Check sheet for the modelled part. Datum: model origin and axes. Units: mm. A direction names the side the tool comes from. Round coordinates to 2 decimals unless told otherwise and drop trailing zeros. Loops run counter-clockwise (first coordinate to the right, second up) from the corner with the lowest first, then second, coordinate; pieces in that order, holes last. Notation, with made-up numbers: (18, 0.5) -> (67, 0.5) arc R24 cw to (67, 13.5) -> close; hole circle Ø3 at (19, 10). An arc over 180 degrees is marked (long way). Return JSON: item names as keys, results as strings.
from build123d import *

# Parameters (mm, degrees)
F0_R     = 11
F1_DEPTH = 6


with BuildPart() as f1:
    # F0 (on Top) → F1 (new body)
    with BuildSketch(Plane.XY):
        with BuildLine():
            Line((11.2187429189, 11.8292181419), (3.5389187623, 33.7403846154))
            ThreePointArc((3.5389187623, 33.7403846154), (0, 36.25), (-3.5389187623, 33.7403846154))
            Line((-3.5389187623, 33.7403846154), (-11.2187429189, 11.8292181419))
            ThreePointArc((-11.2187429189, 11.8292181419), (-13.1608995727, 7.5984489111), (-15.8537748772, 3.8011072954))
            Line((-15.8537748772, 3.8011072954), (-30.9894895915, -13.8053987576))
            ThreePointArc((-30.9894895915, -13.8053987576), (-28.3703151015, -12.5067254343), (-25.6147048476, -13.4830653025))
            ThreePointArc((-25.6147048476, -13.4830653025), (-24.8982303588, -14.375), (-24.4840294966, -15.4414524572))
            ThreePointArc((-24.4840294966, -15.4414524572), (-24.4179418082, -15.8433278187), (-24.395825623, -16.25))
            ThreePointArc((-24.395825623, -16.25), (-25.2588111204, -18.643250355), (-27.4505708292, -19.9349858577))
            Line((-27.4505708292, -19.9349858577), (-4.6350319583, -15.6303254372))
            ThreePointArc((-4.6350319583, -15.6303254372), (0, -15.1968978222), (4.6350319583, -15.6303254372))
            Line((4.6350319583, -15.6303254372), (27.4505708292, -19.9349858577))
            ThreePointArc((27.4505708292, -19.9349858577), (25.016299495, -18.3160508741), (24.4840294966, -15.4414524572))
            ThreePointArc((24.4840294966, -15.4414524572), (24.8982303588, -14.375), (25.6147048476, -13.4830653025))
            ThreePointArc((25.6147048476, -13.4830653025), (28.3703151015, -12.5067254343), (30.9894895915, -13.8053987576))
            Line((30.9894895915, -13.8053987576), (15.8537748772, 3.8011072954))
            ThreePointArc((15.8537748772, 3.8011072954), (13.1608995727, 7.5984489111), (11.2187429189, 11.8292181419))
        make_face()
        with BuildLine():
            Line((-19.4313725784, -12.3734087272), (-12.0274698164, -8.0987634745))
            ThreePointArc((-12.0274698164, -8.0987634745), (-10.1599093098, -10.3453488494), (-7.8799155315, -12.171973185))
            Line((-7.8799155315, -12.171973185), (-18.7459713, -14.2220970264))
            ThreePointArc((-18.7459713, -14.2220970264), (-19.8690053401, -13.5870615238), (-19.4313725784, -12.3734087272))
        make_face(mode=Mode.SUBTRACT)
        with BuildLine():
            ThreePointArc((-20.4313725784, -10.6413579197), (-21.7012431124, -10.4135326105), (-21.68968297, -9.1234388512))
            Line((-21.68968297, -9.1234388512), (-14.4811957581, -0.7382204374))
            ThreePointArc((-14.4811957581, -0.7382204374), (-14.0392895695, -3.6260651377), (-13.0274698164, -6.366712667))
            Line((-13.0274698164, -6.366712667), (-20.4313725784, -10.6413579197))
        make_face(mode=Mode.SUBTRACT)
        with BuildLine():
            ThreePointArc((19.4313725784, -12.3734087272), (19.8690053401, -13.5870615238), (18.7459713, -14.2220970264))
            Line((18.7459713, -14.2220970264), (7.8799155315, -12.171973185))
            ThreePointArc((7.8799155315, -12.171973185), (10.1599093098, -10.3453488494), (12.0274698164, -8.0987634745))
            Line((12.0274698164, -8.0987634745), (19.4313725784, -12.3734087272))
        make_face(mode=Mode.SUBTRACT)
        Circle(F0_R, mode=Mode.SUBTRACT)
        with BuildLine():
            Line((14.4811957581, -0.7382204374), (21.68968297, -9.1234388512))
            ThreePointArc((21.68968297, -9.1234388512), (21.7012431124, -10.4135326105), (20.4313725784, -10.6413579197))
            Line((20.4313725784, -10.6413579197), (13.0274698164, -6.366712667))
            ThreePointArc((13.0274698164, -6.366712667), (14.0392895695, -3.6260651377), (14.4811957581, -0.7382204374))
        make_face(mode=Mode.SUBTRACT)
        with BuildLine():
            Line((-6.6012802267, 12.9101936225), (-2.9437116699, 23.3455358777))
            ThreePointArc((-2.9437116699, 23.3455358777), (-1.8322377723, 24.0005941343), (-1, 23.0147666469))
            Line((-1, 23.0147666469), (-1, 14.4654761415))
            ThreePointArc((-1, 14.4654761415), (-3.8793802597, 13.9714139872), (-6.6012802267, 12.9101936225))
        make_face(mode=Mode.SUBTRACT)
        with BuildLine():
            ThreePointArc((1, 23.0147666469), (1.8322377723, 24.0005941343), (2.9437116699, 23.3455358777))
            Line((2.9437116699, 23.3455358777), (6.6012802267, 12.9101936225))
            ThreePointArc((6.6012802267, 12.9101936225), (3.8793802597, 13.9714139872), (1, 14.4654761415))
            Line((1, 14.4654761415), (1, 23.0147666469))
        make_face(mode=Mode.SUBTRACT)
        with BuildLine():
            ThreePointArc((-25.6147048476, -13.4830653025), (-28.3703151015, -12.5067254343), (-30.9894895915, -13.8053987576))
            ThreePointArc((-30.9894895915, -13.8053987576), (-31.3934208872, -18.125), (-27.4505708292, -19.9349858577))
            ThreePointArc((-27.4505708292, -19.9349858577), (-25.2588111204, -18.643250355), (-24.395825623, -16.25))
            ThreePointArc((-24.395825623, -16.25), (-24.4179418082, -15.8433278187), (-24.4840294966, -15.4414524572))
            ThreePointArc((-24.4840294966, -15.4414524572), (-24.8982303588, -14.375), (-25.6147048476, -13.4830653025))
        make_face()
        with BuildLine():
            ThreePointArc((31.895825623, -16.25), (31.6619484793, -14.9463972771), (30.9894895915, -13.8053987576))
            ThreePointArc((30.9894895915, -13.8053987576), (28.3703151015, -12.5067254343), (25.6147048476, -13.4830653025))
            ThreePointArc((25.6147048476, -13.4830653025), (24.8982303588, -14.375), (24.4840294966, -15.4414524572))
            ThreePointArc((24.4840294966, -15.4414524572), (25.016299495, -18.3160508741), (27.4505708292, -19.9349858577))
            ThreePointArc((27.4505708292, -19.9349858577), (30.539075978, -19.1370145026), (31.895825623, -16.25))
        make_face()
    extrude(amount=F1_DEPTH)


solid = f1.part
Q1. Section check A-A (x = 0). Record the boundary of the cut face in (y, z).
Results list:
{"outline": "(-15.2, 0) -> (-11, 0) -> (-11, 6) -> (-15.2, 6) -> close; (11, 0) -> (36.25, 0) -> (36.25, 6) -> (11, 6) -> close"}
Q2. Draft check along X on faces 1 (the cylindrical face through (13.194, 7.542, 2.958)), 2 (the cylindrical face through (-1.852, 24.004, 2.958)), 3 (the flat face through (-7.325, 22.938, 2.958)). Enter one of: released by +X, released by -X, zero draft, split by the parting line, or undercut.
Results list:
{"face 1": "released by +X", "face 2": "undercut", "face 3": "released by -X"}
Q3. Tool access check on faces 4 (the flat face through (15.88, -17.75, 2.96)), 5 (the cylindrical face through (-19.86, -13.61, 2.96)), 6 (the flat face through (23.53, -5.13, 2.96)). Record the directions out of +Z, -Z, +X, -X, +Y, -Y that give a thin tool (end or side, any length) a straight path to the whole face; none if there is none.
Results list:
{"face 4": "+Z, -Z, -Y", "face 5": "+Z, -Z", "face 6": "+Z, -Z, +X, +Y"}
Q4. Go/stop test with flat-tipped pins: pin 1 (1.5 mm diameter, centred on y = 29.5, z = 5.5, fed in from -X); pin 2 (1 mm diameter, centred on x = 13, z = 4.5, fed in from -Y); pin 3 (17.5 mm diameter, centred on x = 0, y = 0, fed in from -Z). Record where each tip stops, or that it passes through.
Results list:
{"pin 1": "x = -5.29", "pin 2": "y = -17.3", "pin 3": "through"}
Q5. Section check D-D (y = 25). Record the boundary of the cut face in (x, z).
Results list:
{"outline": "(-6.6, 0) -> (6.6, 0) -> (6.6, 6) -> (-6.6, 6) -> close"}
Q6. Section check C-C (z = 5.1). Count the separate pieces of the cut face and the enclosed holes in it, then the cut area to 3 significant figures.
Results list:
{"separate pieces": "1", "enclosed holes": "7", "area": "1,030 mm^2"}
Q7. Material ranges on line 1 (Y direction, x = 0, z = 1.7); line 2 (X direction, y = 18, z = 3.5); line 3 (X direction, y = -4.5, z = 2.15), recorded low to high.
Results list:
{"line 1": "-15.2 to -11, 11 to 36.25", "line 2": "-9.06 to -4.82, -1 to 1, 4.82 to 9.06", "line 3": "-22.99 to -17.72, -13.78 to -10.04, 10.04 to 13.78, 17.72 to 22.99"}
Q8. Section check B-B (y = 0). Record the boundary of the cut face in (x, z), then the cut area to 3 significant figures.
Results list:
{"outline": "(-19.12, 0) -> (-11, 0) -> (-11, 6) -> (-19.12, 6) -> close; (11, 0) -> (19.12, 0) -> (19.12, 6) -> (11, 6) -> close", "area": "97.5 mm^2"}
